Here's how the part is built. I have some questions about the finished solid (model axes, mm). A direction names the side the tool comes from. Give positions to 0.01 mm unless a question says otherwise; leave off trailing zeros. Answer in a Markdown table with one row per item. Add a question column.
Item 1: If we section it at A-A (y = -21.59): Give the number of separate pieces and of enclosed holes in the cut face, then the cut area to 3 significant figures.
Item 2: If I drill on line 1 (X direction, y = -21.59, z = -5.5); line 2 (Z direction, x = 10, y = 42) (3 decimals), over which ranges is the centre line in solid material (lowest first)?
Item 3: For P1, Ø5.5, axis at x = 60.325, y = -21.59, coming from the -Z side; P2, Ø1.4, axis at x = 12.5, y = 13.5, coming from the -Z side, each with a flat end and sliding along its axis, tell me the tip position at first contact or that it passes through.
Item 4: We'd pull the mould along Y, two halves only. Please class faces 1 (the face through (-43, 46.99, 0)), 2 (the face through (-158.75, 1, 0)), 3 (the face through (-146.41, -20.12, -0.13)): released by +Y, released by -Y, zero draft, split by the parting line, or undercut.
Item 5: Which directions (+Z, -Z, +X, -X, +Y, -Y) give clear straight access to the entire face, cutting with the end or side of a thin tool? Please do faces 4 (the face through (57.65, 19.88, -0.13)), 5 (the face through (34, 1, -7.493)).
```python
from build123d import *

# Parameters (mm, degrees)
BOSS_EXTRUDE2_DEPTH = 46.99


with BuildPart() as part:
    # 3DSketch2 → Boss-Extrude2 (new, symmetric)
    with BuildSketch(Plane(origin=(69.85, 0, -9.525), x_dir=(-0.9965457582448797, 0, 0.08304547985373997), z_dir=(0, 1, 0))):
        Polygon((0, 0), (33.222344215, -2.768528685), (33.391092631, -0.743547704), (38.137141804, -1.139051802), (37.968393389, -3.164032782), (55.370573692, -4.614214474), (55.539322108, -2.589233494), (60.285371281, -2.984737591), (60.116622866, -5.009718572), (227.810360335, -18.984196695), (229.392376726, 0), (1.582016391, 18.984196695), align=None)
    extrude(amount=BOSS_EXTRUDE2_DEPTH, both=True)

    # Sketch1 → 1/4 (0.25) Diameter Hole1 (revolve, cut)
    with BuildSketch(Plane(origin=(-149.225, -21.59, -9.525), x_dir=(0, 1, 0), z_dir=(1, 0, 0))):
        Polygon((0, 0), (0, 20.957732465), (3.175, 19.05), (3.175, 0), align=None)
    f_1_4_0_25_diameter_hole1 = revolve(axis=Axis((-149.225, -21.59, -15.875), (0, 0, 1)), mode=Mode.SUBTRACT)

    # Mirror1: 1/4 (0.25) Diameter Hole1 across plane
    add(f_1_4_0_25_diameter_hole1.mirror(Plane.ZX), mode=Mode.SUBTRACT)

    # Sketch3 → 1/4 (0.25) Diameter Hole2 (revolve, cut)
    with BuildSketch(Plane(origin=(60.325, -21.59, -9.525), x_dir=(0, 1, 0), z_dir=(1, 0, 0))):
        Polygon((0, 0), (0, 20.957732465), (3.175, 19.05), (3.175, 0), align=None)
    f_1_4_0_25_diameter_hole2 = revolve(axis=Axis((60.325, -21.59, -15.875), (0, 0, 1)), mode=Mode.SUBTRACT)

    # Mirror2: 1/4 (0.25) Diameter Hole2 across plane
    add(f_1_4_0_25_diameter_hole2.mirror(Plane.ZX), mode=Mode.SUBTRACT)


solid = part.part
```
Recorded:
| question | item | result |
|---|---|---|
| 1 | separate pieces | 3 |
| 1 | enclosed holes | 0 |
| 1 | area | 4,090 mm^2 |
| 2 | line 1 | x = -158.75 to -152.4, -146.05 to 57.15, 63.5 to 69.85 |
| 2 | line 2 | z = -7.493 to 9.525 |
| 3 | P1 | passes through |
| 3 | P2 | stops at z = -7.49 |
| 4 | face 1 | released by +Y |
| 4 | face 2 | zero draft |
| 4 | face 3 | undercut |
| 5 | face 4 | +Z, -Z |
| 5 | face 5 | -Z, +Y, -Y |
